from build123d import *

# Parameters (mm, degrees)
F0_R     = 1.22
F1_DEPTH = 2.4


with BuildPart() as f1:
    # F0 (on Front) → F1 (new body)
    with BuildSketch(Plane.XZ):
        with BuildLine():
            Line((62.29, 21.44), (0, 21.44))
            Line((0, 21.44), (0, 0))
            Line((0, 0), (24.263217, 0))
            Line((24.263217, 0), (36.140737, -29.43386))
            ThreePointArc((36.140737, -29.43386), (58.601735, -8.82154), (62.29, 21.44))
        make_face()
        with Locations((38.522564, -25.937207)):
            Circle(F0_R, mode=Mode.SUBTRACT)
        with Locations((3.840634, 6.738324)):
            Circle(F0_R, mode=Mode.SUBTRACT)
        with Locations((3.680635, 17.136306)):
            Circle(F0_R, mode=Mode.SUBTRACT)
        with Locations((19.822557, 11.133424)):
            Circle(F0_R, mode=Mode.SUBTRACT)
        with Locations((54.667417, 14.196431)):
            Circle(F0_R, mode=Mode.SUBTRACT)
    extrude(amount=F1_DEPTH)


solid = f1.part
Can you work these out from the model? Positions are in its coordinate system, mm. Coordinates: 2 decimals unless noted, no trailing zeros. Loops run counter-clockwise (first coordinate to the right, second up) from the corner with the lowest first, then second, coordinate; pieces in that order, holes last. Notation, with made-up numbers: (76, -28) - (115, -28) arc R5 cw to (115, -20) - close; hole circle Ø3 at (-21, 37.5). An arc over 180 degrees is marked (long way). Put each result on its own line as item: value. Start each with the question number.
Item 1: For pin 1 (2 mm diameter, centred on x = 38.52, z = -25.94, fed in from -Y), with a flat end and sliding along its axis, tell me the tip position at first contact or that it passes through.
Item 2: Suppose I cut it at B-B (y = -0.8). Please give me the cut outline in (x, z).
Item 3: Suppose I cut it at A-A (x = 19.5). Please give me the cut outline in (y, z).
Item 4: If I drill on line 1 along Z through (x, y) = (20, -1.5); line 2 along Z through (x, y) = (24, -2.15); line 3 along Z through (x, y) = (19, -1.4), over which ranges is the centre line in solid material (lowest first)?
Item 5: Suppose I cut it at D-D (x = 51.5). Please give me the cut outline in (y, z).
Item 6: Suppose I cut it at C-C (z = 1.5). Please give me the cut outline in (x, y).
Item 7: If we mould it in two halves opening along X, with no side actions, what happens to faces 1 (the face through (39.086, -1.183, -27.02)), 2 (the face through (0, -1, 11)), 3 (the face through (12, -1, 0))? For each: +X half, -X half, draft (parallel to the pull), parting line (faces both ways), or undercut.
Here are the results:
1. pin 1: through
2. outline: (0, 0) - (24.26, 0) - (36.14, -29.43) arc R44.03 ccw to (62.29, 21.44) - (0, 21.44) - close; hole circle Ø2.44 at (3.68, 17.14); hole circle Ø2.44 at (3.84, 6.74); hole circle Ø2.44 at (19.82, 11.13); hole circle Ø2.44 at (38.52, -25.94); hole circle Ø2.44 at (54.67, 14.2)
3. outline: (-2.4, 0) - (0, 0) - (0, 9.96) - (-2.4, 9.96) - close; (-2.4, 12.31) - (0, 12.31) - (0, 21.44) - (-2.4, 21.44) - close
4. line 1: 0 to 9.93, 12.34 to 21.44
4. line 2: 0 to 21.44
4. line 3: 0 to 10.23, 12.03 to 21.44
5. outline: (-2.4, -18.87) - (0, -18.87) - (0, 21.44) - (-2.4, 21.44) - close
6. outline: (0, -2.4) - (62.37, -2.4) - (62.37, 0) - (0, 0) - close
7. face 1: undercut
7. face 2: -X half
7. face 3: draft
